The model under review builds one solid part; all positions refer to its coordinate system, in mm. A direction names the side the tool comes from. Coordinates: 2 decimals unless noted, no trailing zeros. Write each loop counter-clockwise with the first axis right and the second up, starting at its lowest first coordinate (ties: lowest second). Pieces come first, ordered by that corner, then holes. Notation, with made-up numbers: (-17, 68) - (33, 68) arc R25 ccw to (33, 106) - close; hole circle Ø10 at (1.25, 69). An arc over 180 degrees is marked (long way). Put each result on its own line as item: value. Start each with the question number.
Item 1: Consider section C-C on z = -2.5. Give the boundary of the cut face in (x, y).
Item 2: For pin 1 (4 mm diameter, centred on y = 3.5, z = -9.5, fed in from -X); pin 2 (1.5 mm diameter, centred on y = 2, z = -3, fed in from +X); pin 3 (4 mm diameter, centred on y = -3, z = -2.5, fed in from -X), all flat-tipped, find the tip position at first contact; note any pin that passes through.
Item 3: Machinability: for faces 1 (the face through (0, 0, -27.183)), 2 (the face through (-2.81, 0.89, -4.93)), which of the approach directions +Z, -Z, +X, -X, +Y, -Y give a long, thin tool a straight path to every point of the face, cutting with its end or side? Answer none if there is none.
Item 4: To check wall thickness, follow L1, parallel to Z at x = 4.5, y = -1.5; L2, parallel to Z at x = -0.25, y = 2.25; L3, parallel to Y at x = -0.75, z = -1.5. State the ranges of each line that lie inside material, in increasing order. Write a range as [from, to].
Item 5: Consider section D-D on x = -1.75. Give the boundary of the cut face in (y, z), then the cut area to 3 significant figures.
Item 6: Consider section A-A on x = 0. Give the boundary of the cut face in (y, z).
```python
from build123d import *

# Parameters (mm, degrees)
SKETCH_1_R      = 5
EXTRUDE_1_DEPTH = 3
SKETCH_2_R      = 2.948811386
EXTRUDE_2_DEPTH = 10
SKETCH_3_R      = 1.122261049
EXTRUDE_3_DEPTH = 17.182541617


with BuildPart() as part:
    # 草图1 → 凸台-拉伸1 (new body)
    with BuildSketch(Plane.XY):
        Circle(SKETCH_1_R)
    extrude(amount=EXTRUDE_1_DEPTH)

    # 草图2 → 凸台-拉伸2 (add)
    with BuildSketch(Plane(origin=(0, 0, 0), x_dir=(-1, 0, 0), z_dir=(0, 0, -1))):
        Circle(SKETCH_2_R)
    extrude(amount=EXTRUDE_2_DEPTH)

    # 草图3 → 凸台-拉伸3 (add)
    with BuildSketch(Plane(origin=(0, 0, -10), x_dir=(-1, 0, 0), z_dir=(0, 0, -1))):
        Circle(SKETCH_3_R)
    extrude(amount=EXTRUDE_3_DEPTH)


solid = part.part
```
Report:
1. outline: circle Ø5.9 at (0, 0)
2. pin 1: x = -2.54
2. pin 2: x = 2.67
2. pin 3: x = -2.77
3. face 1: -Z, +X, -X, +Y, -Y
3. face 2: -Z
4. L1: [0, 3]
4. L2: [-10, 3]
4. L3: [-2.85, 2.85]
5. outline: (-4.68, 0) - (-2.37, 0) - (-2.37, -10) - (2.37, -10) - (2.37, 0) - (4.68, 0) - (4.68, 3) - (-4.68, 3) - close
5. area: 75.6 mm²
6. outline: (-5, 0) - (-2.95, 0) - (-2.95, -10) - (-1.12, -10) - (-1.12, -27.18) - (1.12, -27.18) - (1.12, -10) - (2.95, -10) - (2.95, 0) - (5, 0) - (5, 3) - (-5, 3) - close
